For this review, take the finished solid that the model builds, in its own axes (mm). Face numbers are marked on the shaded views. A direction names the side the tool comes from. Round coordinates to 2 decimals unless told otherwise and drop trailing zeros. Write each loop counter-clockwise with the first axis right and the second up, starting at its lowest first coordinate (ties: lowest second). Pieces come first, ordered by that corner, then holes. Notation, with made-up numbers: (87, 20.5) -> (113, 20.5) arc R18 cw to (113, 44.5) -> close; hole circle Ø4 at (85, -9). An arc over 180 degrees is marked (long way). Answer in a Markdown table with one row per item. Add a question column.
```python
from build123d import *

# Parameters (mm, degrees)
BOSS_EXTRUDE1_DEPTH     = 19.05
BOSS_EXTRUDE2_DEPTH     = 95.25
SKETCH4_R               = 2.413
CUT_EXTRUDE1_DEPTH      = 1
CUT_EXTRUDE1_DEPTH_BACK = 39.1
SKETCH5_R               = 2.159
CUT_EXTRUDE2_DEPTH      = 121.6500001
CUT_EXTRUDE2_DEPTH_BACK = 7.35
BOSS_EXTRUDE3_DEPTH     = 3.175
FILLET1_R               = 6.35
FILLET2_R               = 3.175


with BuildPart() as part:
    # Sketch1 → Boss-Extrude1 (new body, symmetric)
    with BuildSketch(Plane.XY):
        Polygon((0, 0), (63.5, 0), (63.5, 127), (57.15, 127), (57.15, 6.35), (0, 6.35), align=None)
    extrude(amount=BOSS_EXTRUDE1_DEPTH, both=True)

    # Sketch3 → Boss-Extrude2 (add)
    with BuildSketch(Plane(origin=(0, 127, 0), x_dir=(1, 0, 0), z_dir=(0, 1, 0))):
        with BuildLine():
            Line((95.25, 19.05), (63.5, 19.05))
            Line((63.5, 19.05), (63.5, -19.05))
            Line((63.5, -19.05), (95.25, -19.05))
            Line((95.25, -19.05), (95.25, -9.525))
            Line((95.25, -9.525), (88.767695047, -9.525))
            ThreePointArc((88.767695047, -9.525), (70.144285562, 0), (88.767695047, 9.525))
            Line((88.767695047, 9.525), (95.25, 9.525))
            Line((95.25, 9.525), (95.25, 19.05))
        make_face()
    extrude(amount=-BOSS_EXTRUDE2_DEPTH)

    # Sketch4 → Cut-Extrude1 (cut, two sides)
    with BuildSketch(Plane.XY.offset(19.05)) as cut_extrude1_sk:
        with Locations((79.375, 105.41)):
            Circle(SKETCH4_R)
        with Locations((79.375, 50.8)):
            Circle(SKETCH4_R)
        with Locations((79.375, 77.47)):
            Circle(SKETCH4_R)
    extrude(amount=CUT_EXTRUDE1_DEPTH, mode=Mode.SUBTRACT)
    extrude(cut_extrude1_sk.sketch, amount=-CUT_EXTRUDE1_DEPTH_BACK, mode=Mode.SUBTRACT)

    # Sketch5 → Cut-Extrude2 (cut, two sides)
    with BuildSketch(Plane(origin=(0, 6.35, 0), x_dir=(1, 0, 0), z_dir=(0, 1, 0))) as cut_extrude2_sk:
        with Locations((12.7, 10.16)):
            Circle(SKETCH5_R)
        with Locations((44.45, -10.16)):
            Circle(SKETCH5_R)
    extrude(amount=CUT_EXTRUDE2_DEPTH, mode=Mode.SUBTRACT)
    extrude(cut_extrude2_sk.sketch, amount=-CUT_EXTRUDE2_DEPTH_BACK, mode=Mode.SUBTRACT)

    # Sketch6 → Boss-Extrude3 (add)
    with BuildSketch(Plane.XY.offset(19.05)):
        Polygon((57.15, 127), (0, 6.35), (57.15, 6.35), align=None)
    boss_extrude3 = extrude(amount=-BOSS_EXTRUDE3_DEPTH)

    # Mirror1: Boss-Extrude3 across plane
    add(boss_extrude3.mirror(Plane.XY))

    # Fillet1
    fillet1_edges = [part.edges().sort_by_distance(p)[0] for p in [
        (57.15, 6.35, 0),
    ]]
    fillet(fillet1_edges, radius=FILLET1_R)

    # Fillet2
    fillet2_edges = [part.edges().sort_by_distance(p)[0] for p in [
        (25.4, 6.35, -15.875),
        (25.4, 6.35, 15.875),
        (55.290128061, 8.209871939, -15.875),
        (55.290128061, 8.209871939, 15.875),
        (57.15, 69.85, 15.875),
        (57.15, 69.85, -15.875),
    ]]
    fillet(fillet2_edges, radius=FILLET2_R)


solid = part.part
```
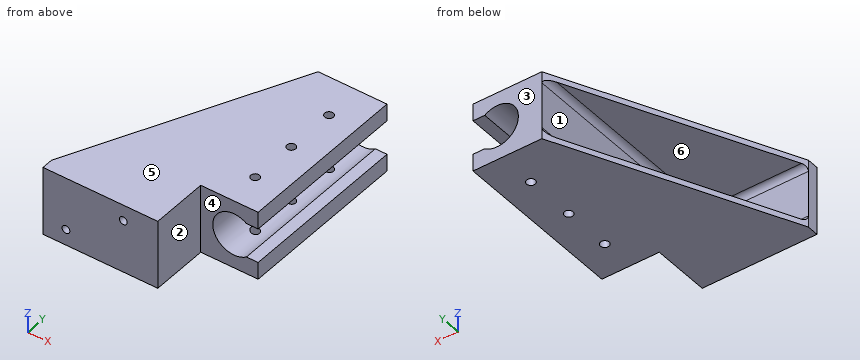
1. We need section C-C (x = 86.5). Write out the cut boundary in (y, z), plus the area to 3 significant figures.
2. For L1, parallel to Z at x = 27, y = 48 (3 decimals); L2, parallel to X at y = 2.25, z = -10.16; L3, parallel to Y at x = 64, z = 3.5, list the stretches that pass through material, from the lowest coordinate up. Write a range as [from, to].
3. Clearance check with flat-ended pins moving along their axes: pin 1 Ø4 at (x, z) = (75, -8) entering from -Y; pin 2 Ø7 at (x, z) = (12.7, -10.16) entering from +Y; pin 3 Ø7.5 at (x, z) = (31.5, -0.5) entering from +Y; pin 4 Ø3 at (x, y) = (12.5, 33) entering from +Z. State where each tip first meets the part, or that it passes through.
4. We need section A-A (y = 105.41). Count the separate pieces of the cut face and the enclosed holes in it, plus the area to 3 significant figures.
5. We need section D-D (z = 0). Write out the cut boundary in (x, y), plus the area to 3 significant figures.
6. Tool access review of the marked faces 1, 2 and 3: name each direction out of +Z, -Z, +X, -X, +Y, -Y from which nothing blocks a thin tool from reaching the whole face with its end or side.
7. The part is to be moulded in two halves that separate along Z. For the marked faces 4, 5 and 6, say which applies: pulls with the +Z half, pulls with the -Z half, needs draft (parallel to the pull), parting line crosses it, or undercut.
8. We need section B-B (x = 27). Write out the cut boundary in (y, z) (3 decimals).
Response:
| question | item | result |
|---|---|---|
| 1 | outline | (31.75, -19.05) -> (127, -19.05) -> (127, -10.81) -> (31.75, -10.81) -> close; (31.75, 10.81) -> (127, 10.81) -> (127, 19.05) -> (31.75, 19.05) -> close |
| 1 | area | 1,570 mm2 |
| 2 | L1 | [-19.05, -15.875], [15.875, 19.05] |
| 2 | L2 | [0, 10.54], [14.86, 63.5] |
| 2 | L3 | [31.75, 127] |
| 3 | pin 1 | y = 31.75 |
| 3 | pin 2 | y = 6.5 |
| 3 | pin 3 | y = 6.35 |
| 3 | pin 4 | z = 19.05 |
| 4 | separate pieces | 3 |
| 4 | enclosed holes | 0 |
| 4 | area | 955 mm2 |
| 5 | outline | (0, 0) -> (63.5, 0) -> (63.5, 31.75) -> (70.14, 31.75) -> (70.14, 127) -> (57.15, 127) -> (57.15, 12.7) arc R6.35 cw to (50.8, 6.35) -> (0, 6.35) -> close |
| 5 | area | 1,810 mm2 |
| 6 | face 1 | -X, +Y |
| 6 | face 2 | +Z, -Z, +X, -Y |
| 6 | face 3 | +Z, -Z, +X, -X, +Y |
| 7 | face 4 | needs draft |
| 7 | face 5 | pulls with the +Z half |
| 7 | face 6 | undercut |
| 8 | outline | (0, -19.05) -> (63.35, -19.05) -> (63.35, -15.875) -> (9.525, -15.875) arc R3.175 cw to (6.35, -12.7) -> (6.35, 12.7) arc R3.175 cw to (9.525, 15.875) -> (63.35, 15.875) -> (63.35, 19.05) -> (0, 19.05) -> close |
